```python
from build123d import *

# Parameters (mm, degrees)
SKETCH1_W           = 9
SKETCH1_H           = 9
BOSS_EXTRUDE1_DEPTH = 5
SKETCH2_R           = 1.6
CUT_EXTRUDE1_DEPTH  = 4.5
SKETCH3_R           = 1.6
CUT_EXTRUDE2_DEPTH  = 4.5
SKETCH4_R           = 1.6
CUT_EXTRUDE3_DEPTH  = 4.5
CHAMFER1_SIZE       = 1.1
CHAMFER2_SIZE       = 5
CHAMFER3_SIZE       = 0.4


with BuildPart() as part:
    # Sketch1 → Boss-Extrude1 (new body)
    with BuildSketch(Plane.XY):
        Rectangle(SKETCH1_W, SKETCH1_H)
    extrude(amount=BOSS_EXTRUDE1_DEPTH)

    # Sketch2 → Cut-Extrude1 (cut)
    with BuildSketch(Plane(origin=(0, 0, 0), x_dir=(-1, 0, 0), z_dir=(0, 0, -1))):
        with Locations((-2, -2)):
            Circle(SKETCH2_R)
    extrude(amount=-CUT_EXTRUDE1_DEPTH, mode=Mode.SUBTRACT)

    # Sketch3 → Cut-Extrude2 (cut)
    with BuildSketch(Plane(origin=(4.5, 0, 0), x_dir=(0, 0, -1), z_dir=(1, 0, 0))):
        with Locations((-2.5, 2)):
            Circle(SKETCH3_R)
    extrude(amount=-CUT_EXTRUDE2_DEPTH, mode=Mode.SUBTRACT)

    # Sketch4 → Cut-Extrude3 (cut)
    with BuildSketch(Plane.XZ.offset(4.5)):
        with Locations((-2, 2.5)):
            Circle(SKETCH4_R)
    extrude(amount=-CUT_EXTRUDE3_DEPTH, mode=Mode.SUBTRACT)

    # Chamfer1
    chamfer1_edges = [part.edges().sort_by_distance(p)[0] for p in [
        (4.5, -4.5, 2.5),
    ]]
    chamfer(chamfer1_edges, length=CHAMFER1_SIZE)

    # Chamfer2
    chamfer2_edges = [part.edges().sort_by_distance(p)[0] for p in [
        (-4.5, 4.5, 2.5),
    ]]
    chamfer(chamfer2_edges, length=CHAMFER2_SIZE)

    # Chamfer3
    chamfer3_edges = [part.edges().sort_by_distance(p)[0] for p in [
        (4.5, 0.55, 5),
        (3.95, -3.95, 5),
        (-0.55, -4.5, 5),
    ]]
    chamfer(chamfer3_edges, length=CHAMFER3_SIZE)


solid = part.part
```
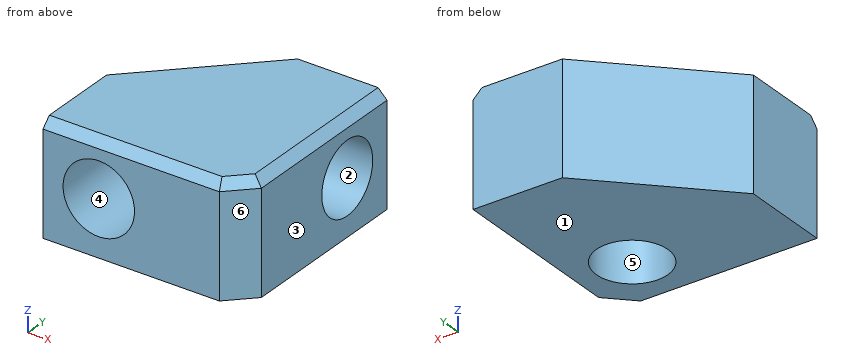
For this review, take the finished solid that the model builds, in its own axes (mm). Face numbers are marked on the shaded views. A direction names the side the tool comes from. Round coordinates to 2 decimals unless told otherwise and drop trailing zeros. Loops run counter-clockwise (first coordinate to the right, second up) from the corner with the lowest first, then second, coordinate; pieces in that order, holes last.
(1) We need section C-C (y = 2). Give the boundary of the cut face in (x, z), plus the area to 3 significant figures.
Returned:
outline: (-2, 0) - (4.5, 0) - (4.5, 0.9) - (0, 0.9) - (0, 4.1) - (4.5, 4.1) - (4.5, 4.6) - (4.1, 5) - (-2, 5) - close
area: 18.0 mm2
(2) We need section A-A (y = -2). Give the boundary of the cut face in (x, z), plus the area to 3 significant figures.
Returned:
outline: (-4.5, 0) - (0.4, 0) - (0.4, 4.5) - (3.6, 4.5) - (3.6, 0) - (4.5, 0) - (4.5, 4.6) - (4.1, 5) - (-4.5, 5) - close; hole circle Ø3.2 at (-2, 2.5)
area: 22.5 mm2
(3) Mouldability with a two-part tool opening along Z and no side actions: class the marked faces 1, 2, 3 and 4 as released by +Z, released by -Z, zero draft, split by the parting line, or undercut.
Returned:
face 1: released by -Z
face 2: undercut
face 3: zero draft
face 4: undercut
(4) Wall thickness on line 1 along Y through (x, z) = (1.95, 2.5); line 2 along X through (y, z) = (-2.75, 2.05); line 3 along Z through (x, y) = (-2, -2.75): over which ranges is each line inside the solid? List them lowest first.
Returned:
line 1: y = -4.5 to -3.6, -0.4 to 0.4, 3.6 to 4.5
line 2: x = -4.5 to -3.54, -0.46 to 0.59, 3.41 to 4.5
line 3: z = 0 to 0.9, 4.1 to 5
(5) Clearance check with a flat-ended pin moving along its axis: P1, Ø3.5, axis at x = 2.5, y = -2.5, coming from the -Z side. State where the tip first meets the part, or that it passes through.
Returned:
P1: stops at z = 0
(6) We need section B-B (x = 2). Give the boundary of the cut face in (y, z), plus the area to 3 significant figures.
Returned:
outline: (-4.5, 0) - (-3.6, 0) - (-3.6, 4.5) - (-0.4, 4.5) - (-0.4, 0) - (4.5, 0) - (4.5, 5) - (-4.1, 5) - (-4.5, 4.6) - close; hole circle Ø3.2 at (2, 2.5)
area: 22.5 mm2
(7) Tool access review of the marked faces 5 and 6: name each direction out of +Z, -Z, +X, -X, +Y, -Y from which nothing blocks a thin tool from reaching the whole face with its end or side.
Returned:
face 5: -Z
face 6: +Z, -Z, +X, -Y
(8) We need section D-D (z = 3.65). Give the boundary of the cut face in (x, y), plus the area to 3 significant figures.
Returned:
outline: (-4.5, -4.5) - (-3.11, -4.5) - (-3.11, 0) - (-0.89, 0) - (-0.89, -4.5) - (3.4, -4.5) - (4.5, -3.4) - (4.5, 0.89) - (0, 0.89) - (0, 3.11) - (4.5, 3.11) - (4.5, 4.5) - (0.5, 4.5) - (-4.5, -0.5) - close; hole circle Ø3.2 at (2, -2)
area: 39.8 mm2
